The model under review builds one solid part; all positions refer to its coordinate system, in mm. A direction names the side the tool comes from. Round coordinates to 2 decimals unless told otherwise and drop trailing zeros. Write each loop counter-clockwise with the first axis right and the second up, starting at its lowest first coordinate (ties: lowest second). Pieces come first, ordered by that corner, then holes.
Item 1: Add section B-B (y = 13.5). Give the boundary of the cut face in (x, z) (3 decimals).
Item 2: Add section D-D (y = 7). Give the boundary of the cut face in (x, z) (3 decimals).
Item 3: Clearance check with flat-ended pins moving along their axes: pin 1 Ø4 at (y, z) = (15, 6) entering from -X; pin 2 Ø1.7 at (x, y) = (0, 7) entering from -Z; pin 3 Ø1.1 at (x, z) = (0, 0) entering from +Y; pin 4 Ø6 at (y, z) = (6.5, -4.5) entering from -X. State where each tip first meets the part, or that it passes through.
Item 4: Add section C-C (z = -4.5). Give the boundary of the cut face in (x, y).
Item 5: Machinability: for faces 4 (the face through (0.993, 6.588, -2.742)), 5 (the face through (0, 14, 3.25)), 6 (the face through (0, 8.5, -5.7)), 7 (the face through (-1.125, 14, 3)), 8 (the face through (0, 5, 1.2)), which of the approach directions +Z, -Z, +X, -X, +Y, -Y give a long, thin tool a straight path to every point of the face, cutting with its end or side? Answer none if there is none.
Item 6: To check wall thickness, follow L1, parallel to Z at x = 0, y = 5.25 (3 decimals); L2, parallel to Z at x = 0, y = 2 (3 decimals); L3, parallel to Y at x = 0, z = -2.9 (3 decimals). State the ranges of each line that lie inside material, in increasing order.
Item 7: Add section A-A (y = 9.5). Give the boundary of the cut face in (x, z) (3 decimals).
Item 8: Draft analysis for pull direction Y (two halves, no side actions). For faces 1 (the face through (0, 10, -1)), 2 (the face through (1.125, 14, 3)), 3 (the face through (-0.23, 5.95, -6.84)), state which applies: +Y half, -Y half, draft (parallel to the pull), parting line (faces both ways), or undercut.
```python
from build123d import *

# Parameters (mm, degrees)
SKETCH1_R           = 8
BOSS_EXTRUDE1_DEPTH = 10
SKETCH2_R           = 1.075
CUT_EXTRUDE1_DEPTH  = 9
SKETCH4_R           = 2.275
CUT_EXTRUDE4_DEPTH  = 11.0000001
SKETCH7_R           = 8
BOSS_EXTRUDE3_DEPTH = 1
SKETCH8_R           = 2.625
SKETCH8_W           = 2.25
SKETCH8_H           = 1.25
BOSS_EXTRUDE4_DEPTH = 6.5
SKETCH9_R           = 1.075
CUT_EXTRUDE5_DEPTH  = 6
CUT_EXTRUDE2_START  = -3.5
CUT_EXTRUDE2_DEPTH  = 2.2
SKETCH10_W          = 3.9924405
SKETCH10_H          = 2.148230377
BOSS_EXTRUDE5_DEPTH = 10


with BuildPart() as part:
    # Sketch1 → Boss-Extrude1 (new body)
    with BuildSketch(Plane(origin=(0, 0, 0), x_dir=(1, 0, 0), z_dir=(0, 1, 0))):
        Circle(SKETCH1_R)
    extrude(amount=BOSS_EXTRUDE1_DEPTH)

    # Sketch2 → Cut-Extrude1 (cut, through all)
    with BuildSketch(Plane.XY):
        with Locations((0, 7)):
            Circle(SKETCH2_R)
    extrude(amount=-CUT_EXTRUDE1_DEPTH, mode=Mode.SUBTRACT)

    # Sketch4 → Cut-Extrude4 (cut, through all)
    with BuildSketch(Plane(origin=(0, 0, 0), x_dir=(1, 0, 0), z_dir=(0, 1, 0))):
        Circle(SKETCH4_R)
    extrude(amount=CUT_EXTRUDE4_DEPTH, mode=Mode.SUBTRACT)

    # Sketch7 → Boss-Extrude3 (add)
    with BuildSketch(Plane(origin=(0, 10, 0), x_dir=(1, 0, 0), z_dir=(0, 1, 0))):
        Circle(SKETCH7_R)
    extrude(amount=BOSS_EXTRUDE3_DEPTH)

    # Sketch8 → Boss-Extrude4 (add)
    with BuildSketch(Plane(origin=(0, 11, 0), x_dir=(1, 0, 0), z_dir=(0, 1, 0))):
        Circle(SKETCH8_R)
        with Locations((0, -2.625)):
            Rectangle(SKETCH8_W, SKETCH8_H)
    extrude(amount=BOSS_EXTRUDE4_DEPTH)

    # Sketch9 → Cut-Extrude5 (cut)
    with BuildSketch(Plane(origin=(0, 17.5, 0), x_dir=(1, 0, 0), z_dir=(0, 1, 0))):
        Circle(SKETCH9_R)
    extrude(amount=-CUT_EXTRUDE5_DEPTH, mode=Mode.SUBTRACT)

    # Sketch3 → Cut-Extrude2 (cut)
    with BuildSketch(Plane.XY.offset(CUT_EXTRUDE2_START)):
        Polygon((0, 4.401923789), (2.25, 5.700961894), (2.25, 8.299038106), (2.25, 11.472802467), (-2.25, 11.472802467), (-2.25, 8.299038106), (-2.25, 5.700961894), align=None)
    extrude(amount=-CUT_EXTRUDE2_DEPTH, mode=Mode.SUBTRACT)

    # Sketch10 → Boss-Extrude5 (add)
    with BuildSketch(Plane.XZ):
        with Locations((-0.06344375, 2.274115189)):
            Rectangle(SKETCH10_W, SKETCH10_H)
    extrude(amount=-BOSS_EXTRUDE5_DEPTH)


solid = part.part
```
Numbers:
1. outline: (-1.125, 2.372) arc R2.625 ccw (long way) to (1.125, 2.372) - (1.125, 3.25) - (-1.125, 3.25) - close; hole circle Ø2.15 at (0, 0)
2. outline: (-2.25, -5.7) - (-2.25, -3.5) - (-1.075, -3.5) - (-1.075, -2.005) arc R2.275 cw to (-1.933, 1.2) - (1.933, 1.2) arc R2.275 cw to (1.075, -2.005) - (1.075, -3.5) - (2.25, -3.5) - (2.25, -5.7) - (1.075, -5.7) - (1.075, -7.927) arc R8 ccw (long way) to (-1.075, -7.927) - (-1.075, -5.7) - close
3. pin 1: passes through
3. pin 2: stops at z = 1.2
3. pin 3: stops at y = 11.5
3. pin 4: stops at x = -7.86
4. outline: (-6.61, 0) - (6.61, 0) - (6.61, 11) - (2.25, 11) - (2.25, 5.7) - (0, 4.4) - (-2.25, 5.7) - (-2.25, 11) - (-6.61, 11) - close
5. face 4: -Z
5. face 5: +Z, +X, -X, +Y
5. face 6: +Y
5. face 7: +Z, -X, +Y
5. face 8: -Y
6. L1: z = -8 to -5.7, -3.5 to -2.275, 1.2 to 8
6. L2: z = -8 to -2.275, 1.2 to 8
6. L3: y = 0 to 5.925, 8.075 to 11
7. outline: circle Ø16 at (0, 0); hole (-2.25, -5.7) - (2.25, -5.7) - (2.25, -3.5) - (-2.25, -3.5) - close; hole (-1.933, 1.2) arc R2.275 ccw (long way) to (1.933, 1.2) - close
8. face 1: -Y half
8. face 2: draft
8. face 3: undercut
